Print and shaded views of the part. All mm, measured from the part's lowest x, y and z. Give positions to 0.01 mm unless a question says otherwise; leave off trailing zeros. Write each loop counter-clockwise with the first axis right and the second up, starting at its lowest first coordinate (ties: lowest second). Pieces come first, ordered by that corner, then holes. Notation, with made-up numbers: (20.5, 40.5) -> (25.5, 40.5) arc R21 cw to (25.5, 69.5) -> close; hole circle Ø5 at (88, -12.75). An arc over 180 degrees is marked (long way). Put each result on its own line as item: value.
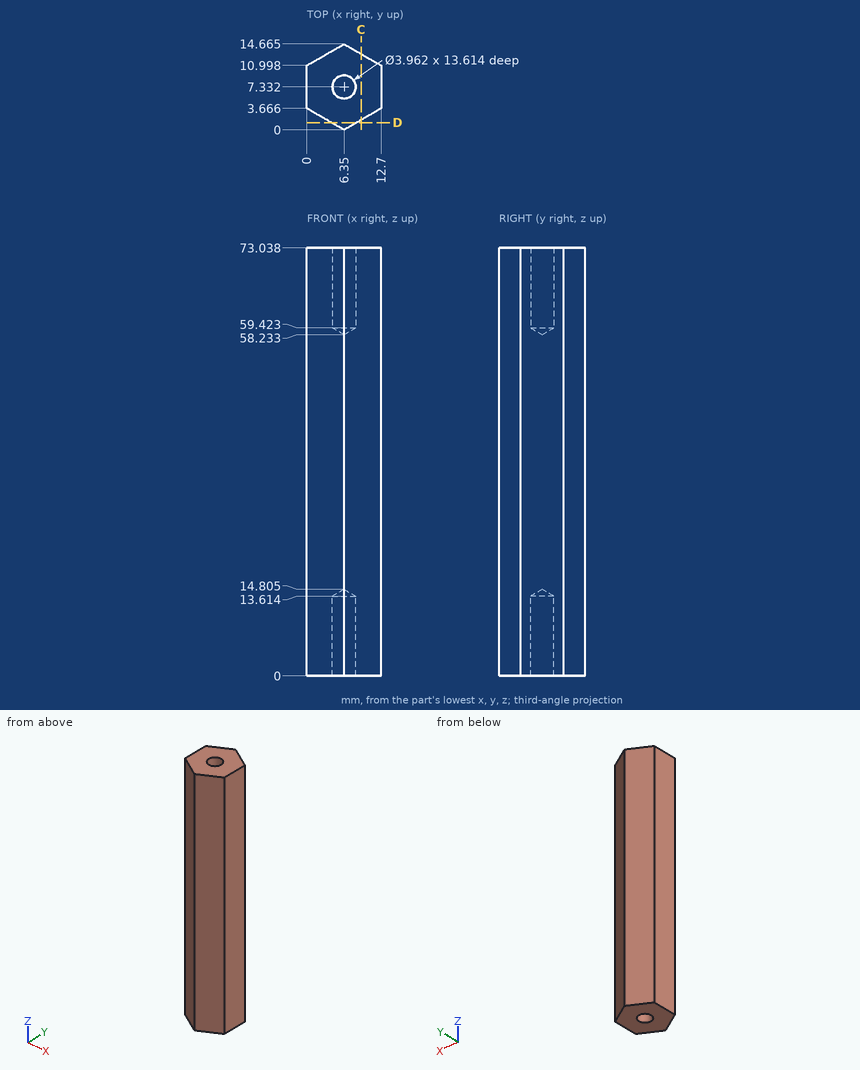
1) Wall check: L1, parallel to X at y = 8.5, z = 11.5; L2, parallel to Z at x = 5.5, y = 8 (1 decimal); L3, parallel to Y at x = 8.5, z = 38 (1 decimal). Give the ranges that are in metal, low to high.
Filled sheet:
L1: 0 to 4.75, 7.95 to 12.7
L2: 14.2 to 58.9
L3: 1.2 to 13.4
2) Slice it at C-C (x = 9.25). Write the cut outline in (y, z) (1 decimal).
Filled sheet:
outline: (1.7, 0) -> (13, 0) -> (13, 73) -> (1.7, 73) -> close
3) Slice it at D-D (y = 1.25). Write the cut outline in (x, z) (1 decimal).
Filled sheet:
outline: (4.2, 0) -> (8.5, 0) -> (8.5, 73) -> (4.2, 73) -> close
